Geometry check sheet. Reference: the model listing, model coordinates, mm. A direction names the side the tool comes from. Coordinates: 2 decimals unless noted, no trailing zeros. Order: outer loops, then holes, each group sorted by start corner. A loop starts at its lowest first (then second) coordinate and runs counter-clockwise, first axis right, second up. Notation, with made-up numbers: (-7.5, 74.25) - (25.5, 74.25) arc R18 ccw to (25.5, 100.25) - close; hole circle Ø3 at (33.25, 29.5). An arc over 180 degrees is marked (long way). Put each result on its own line as item: value.
from build123d import *

# Parameters (mm, degrees)
EXTRUDE_1_DEPTH     = 15
SKETCH_3_R          = 2.5
EXTRUDE_2_DEPTH     = 1
CUT_EXTRUDE_1_DEPTH = 2
EXTRUDE_3_DEPTH     = 9
SKETCH_7_R          = 2
EXTRUDE_4_DEPTH     = 1
EXTRUDE_5_DEPTH     = 10


with BuildPart() as part:
    # 草图1 → 凸台-拉伸1 (new body)
    with BuildSketch(Plane.XY):
        with BuildLine():
            Line((-3.31662479, 0), (3.31662479, 0))
            ThreePointArc((3.31662479, 0), (6, 5), (3.31662479, 10))
            Line((3.31662479, 10), (-3.31662479, 10))
            ThreePointArc((-3.31662479, 10), (-6, 5), (-3.31662479, 0))
        make_face()
    extrude(amount=EXTRUDE_1_DEPTH)

    # 草图3 → 凸台-拉伸2 (add)
    with BuildSketch(Plane.XY):
        with Locations((0, 5)):
            Circle(SKETCH_3_R)
    extrude(amount=-EXTRUDE_2_DEPTH)

    # 草图4 → 切除-拉伸1 (cut)
    with BuildSketch(Plane.XY):
        with BuildLine():
            Line((5, 6), (5.916079783, 6))
            ThreePointArc((5.916079783, 6), (6, 5), (5.916079783, 4))
            Line((5.916079783, 4), (5, 4))
            Line((5, 4), (5, 5))
            Line((5, 5), (5, 6))
        make_face()
        with BuildLine():
            Line((-5, 4), (-5.916079783, 4))
            ThreePointArc((-5.916079783, 4), (-6, 5), (-5.916079783, 6))
            Line((-5.916079783, 6), (-5, 6))
            Line((-5, 6), (-5, 5))
            Line((-5, 5), (-5, 4))
        make_face()
    extrude(amount=CUT_EXTRUDE_1_DEPTH, mode=Mode.SUBTRACT)

    # 草图6 → 凸台-拉伸3 (add)
    with BuildSketch(Plane.XY.offset(15)):
        Polygon((0, 0), (6, 0), (6, 5), (6, 10), (-6, 10), (-6, 5), (-6, 0), align=None)
    extrude(amount=EXTRUDE_3_DEPTH)

    # 草图7 → 凸台-拉伸4 (add)
    with BuildSketch(Plane.XY.offset(24)):
        with Locations((0, 5)):
            Circle(SKETCH_7_R)
    extrude(amount=EXTRUDE_4_DEPTH)

    # 草图8 → 凸台-拉伸5 (add)
    with BuildSketch(Plane.XY.offset(25)):
        with BuildLine():
            Line((1.118033989, 6), (0, 6))
            Line((0, 6), (-1.118033989, 6))
            ThreePointArc((-1.118033989, 6), (-0.535233135, 3.598741462), (1.5, 5))
            ThreePointArc((1.5, 5), (1.401258538, 5.535233135), (1.118033989, 6))
        make_face()
    extrude(amount=EXTRUDE_5_DEPTH)


solid = part.part
Q1. Depth check by flat-ended pin: pin 1 Ø3 at (x, y) = (4.5, 3) entering from -Z; pin 2 Ø0.5 at (x, y) = (-5.5, 5.5) entering from -Z; pin 3 Ø1 at (x, z) = (-5.5, 1) entering from +Y; pin 4 Ø1.5 at (y, z) = (2, 26) entering from -X. Enter the tip coordinate at first touch or a pass-through.
Answer block:
pin 1: stops at z = 0
pin 2: stops at z = 2
pin 3: stops at y = 8.32
pin 4: passes through
Q2. Draft check along Y on faces 4 (the flat face through (0, 6.4, 25)), 5 (the flat face through (5.5, 5, 2)), 6 (the cylindrical face through (-0.26, 6.983, 24.493)). Enter one of: pulls with the +Y half, pulls with the -Y half, needs draft (parallel to the pull), parting line crosses it, or undercut.
Answer block:
face 4: needs draft
face 5: undercut
face 6: parting line crosses it
Q3. Section check C-C on z = 29.5. Record the boundary of the cut face in (x, y).
Answer block:
outline: (-1.12, 6) arc R1.5 ccw (long way) to (1.12, 6) - close
Q4. Thickness scan on L1, parallel to Z at x = -0.75, y = 6.25; L2, parallel to Z at x = 1.5, y = 3.25; L3, parallel to X at y = 1.25, z = 8. Record the ranges inside material, lowest first. Write a range as [from, to].
Answer block:
L1: z = [-1, 25]
L2: z = [-1, 24]
L3: x = [-4.68, 4.68]
Q5. Section check D-D on x = 3.75. Record the boundary of the cut face in (y, z).
Answer block:
outline: (0, 15) - (0.32, 15) - (0.32, 0) - (9.68, 0) - (9.68, 15) - (10, 15) - (10, 24) - (0, 24) - close
Q6. Section check B-B on y = 8. Record the boundary of the cut face in (x, z), then the cut area to 3 significant figures.
Answer block:
outline: (-6, 15) - (-5.2, 15) - (-5.2, 0) - (5.2, 0) - (5.2, 15) - (6, 15) - (6, 24) - (-6, 24) - close
area: 264 mm^2
Q7. Section check A-A on x = 0. Record the boundary of the cut face in (y, z), then the cut area to 3 significant figures.
Answer block:
outline: (0, 0) - (2.5, 0) - (2.5, -1) - (7.5, -1) - (7.5, 0) - (10, 0) - (10, 24) - (7, 24) - (7, 25) - (6, 25) - (6, 35) - (3.5, 35) - (3.5, 25) - (3, 25) - (3, 24) - (0, 24) - close
area: 274 mm^2
Q8. Access from +Z, -Z, +X, -X, +Y, -Y to the whole of each face (thin tool, end or side, straight path). Record for faces 1 (the cylindrical face through (-6, 5, 7)), 2 (the flat face through (0, 6, 30)), 3 (the flat face through (-5, 1, 15)).
Answer block:
face 1: -Z, -X
face 2: +Z, +X, -X, +Y
face 3: -Z, -X, -Y
